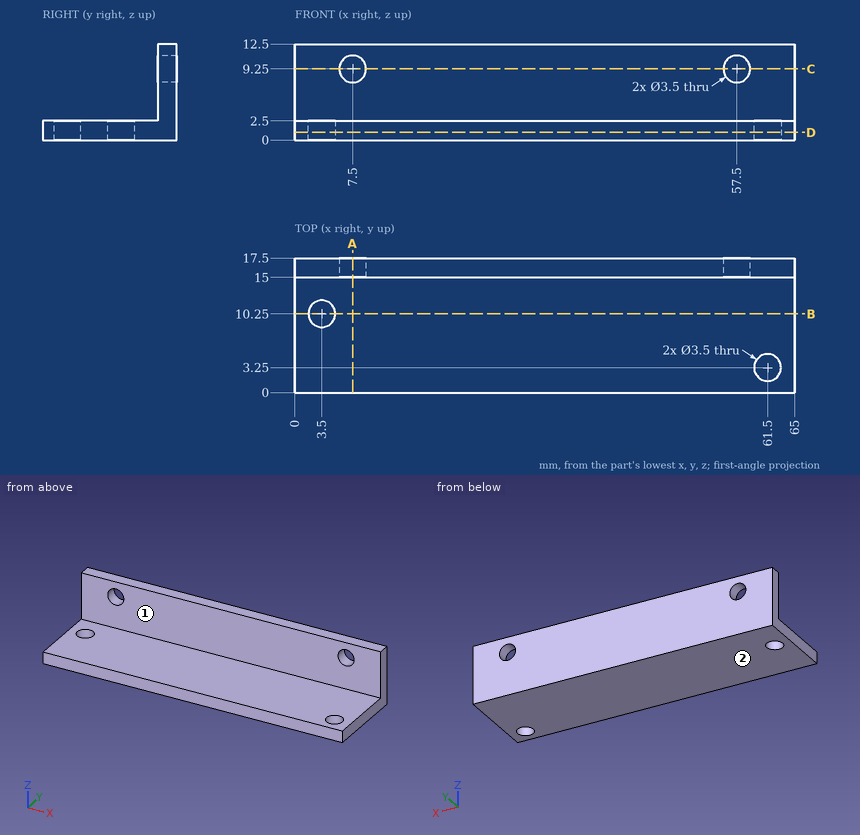
For this review, use the dimensioned drawing (mm, ordinates from the lowest corner) and the shaded views. A direction names the side the tool comes from. Round coordinates to 2 decimals unless told otherwise and drop trailing zeros. Loops run counter-clockwise (first coordinate to the right, second up) from the corner with the lowest first, then second, coordinate; pieces in that order, holes last. Notation, with made-up numbers: M 76,78.5 L 89,78.5 A33 ccw 89,107.5 Z; hole C 51.25,86.5 d1. An arc over 180 degrees is marked long. Answer as a JSON object with one key per item and string values.
(1) Clearance check with flat-ended pins moving along their axes: P1, Ø2, axis at x = 32, z = 10.5, coming from the -Y side; P2, Ø3, axis at x = 29.5, y = 8.5, coming from the +Z side; P3, Ø2, axis at x = 3.5, y = 10.25, coming from the +Z side. State where each tip first meets the part, or that it passes through.
Resolved:
{"P1": "y = 15", "P2": "z = 2.5", "P3": "through"}
(2) To check wall thickness, follow line 1 along Y through (x, z) = (61.5, 1.5); line 2 along Y through (x, z) = (49, 11); line 3 along Z through (x, y) = (61, 8.75). State the ranges of each line that lie inside material, in increasing order.
Resolved:
{"line 1": "0 to 1.5, 5 to 17.5", "line 2": "15 to 17.5", "line 3": "0 to 2.5"}
(3) Take a section at B-B on y = 10.25. Give the boundary of the cut face in (x, z).
Resolved:
{"outline": "M 0,0 L 1.75,0 L 1.75,2.5 L 0,2.5 Z; M 5.25,0 L 65,0 L 65,2.5 L 5.25,2.5 Z"}
(4) Tool access review of the marked faces 1 and 2: name each direction out of +Z, -Z, +X, -X, +Y, -Y from which nothing blocks a thin tool from reaching the whole face with its end or side.
Resolved:
{"face 1": "+Z, +X, -X, -Y", "face 2": "-Z, +X, -X, +Y, -Y"}
(5) Take a section at C-C on z = 9.25. Give the boundary of the cut face in (x, y).
Resolved:
{"outline": "M 0,15 L 5.75,15 L 5.75,17.5 L 0,17.5 Z; M 9.25,15 L 55.75,15 L 55.75,17.5 L 9.25,17.5 Z; M 59.25,15 L 65,15 L 65,17.5 L 59.25,17.5 Z"}
(6) Take a section at A-A on x = 7.5. Give the boundary of the cut face in (y, z), and give its area (3 significant figures).
Resolved:
{"outline": "M 0,0 L 17.5,0 L 17.5,7.5 L 15,7.5 L 15,2.5 L 0,2.5 Z; M 15,11 L 17.5,11 L 17.5,12.5 L 15,12.5 Z", "area": "60.0 mm²"}
(7) Take a section at D-D on z = 1. Give the boundary of the cut face in (x, y).
Resolved:
{"outline": "M 0,0 L 65,0 L 65,17.5 L 0,17.5 Z; hole C 3.5,10.25 d3.5; hole C 61.5,3.25 d3.5"}
